The model under review builds one solid part; all positions refer to its coordinate system, in mm. Face numbers are marked on the shaded views. A direction names the side the tool comes from. Coordinates: 2 decimals unless noted, no trailing zeros. Write each loop counter-clockwise with the first axis right and the second up, starting at its lowest first coordinate (ties: lowest second). Pieces come first, ordered by that corner, then holes. Notation, with made-up numbers: (51, -23) - (97, -23) arc R13 ccw to (97, -12) - close; hole circle Ø6 at (34, -7.75). An arc over 180 degrees is marked (long way). Return JSON: item names as keys, results as strings. Group by question number.
(1) We need section C-C on y = -15.5. State the section outline as (x, z) points.
(2) We need section D-D on z = -16. State the section outline as (x, y) points.
(3) Draft analysis for pull direction X (two halves, no side actions). For the marked faces 4, 5, 6 and 7, state which applies: released by +X, released by -X, zero draft, split by the parting line, or undercut.
(4) We need section A-A on y = -43. State the section outline as (x, z) points.
(5) To check wall thickness, follow L1, parallel to Y at x = 0, z = -1.75; L2, parallel to Y at x = 34, z = 1.5; L3, parallel to Z at x = -31, y = -47. State the ranges of each line that lie inside material, in increasing order. Write a range as from..to.
(6) Tool access review of the marked faces 1, 2 and 3: name each direction out of +Z, -Z, +X, -X, +Y, -Y from which nothing blocks a thin tool from reaching the whole face with its end or side.
(7) For pin 1 Ø1.5 at (x, y) = (37, -30) entering from +Z; pin 2 Ø6 at (x, y) = (10.5, -14) entering from -Z; pin 3 Ø11.5 at (x, z) = (-12, 14) entering from -Y; pin 4 Ø17.5 at (x, y) = (0, -49.53) entering from +Z, all flat-tipped, find the tip position at first contact; note any pin that passes through.
(8) We need section B-B on x = 0. State the section outline as (y, z) points.
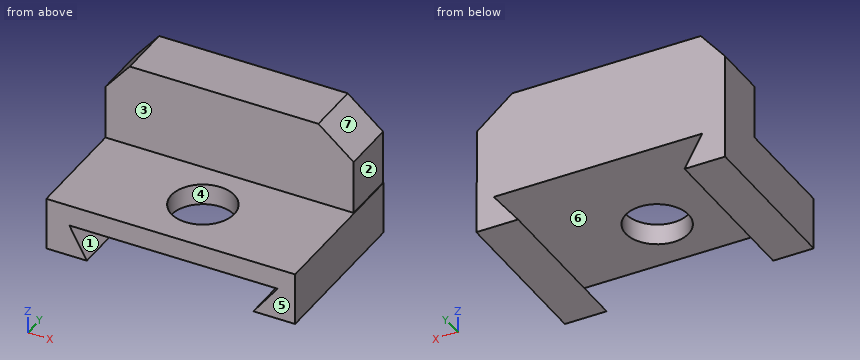
```python
from build123d import *

# Parameters (mm, degrees)
F1_DEPTH = 76.454
F3_DEPTH = 25.4
F4_R     = 14.704348
F5_DEPTH = 25.4


with BuildPart() as f1:
    # F0 (on Front) → F1 (new body)
    with BuildSketch(Plane.XZ):
        Polygon((57.71213, 0), (-58.586556, 0), (-58.586556, -24.629673), (-39.640658, -24.629673), (-47.801968, -9.764426), (49.55082, -9.764426), (38.183279, -24.629673), (57.71213, -24.629673), align=None)
    extrude(amount=F1_DEPTH)

    # F2 (on Front) → F3 (join)
    with BuildSketch(Plane.XZ):
        Polygon((-58.586556, 25.212623), (-58.586556, 0), (57.420652, 0), (57.420652, 25.212623), (40.911183, 38.911968), (-47.219016, 38.911968), align=None)
    extrude(amount=F3_DEPTH)

    # F4 (on Top) → F5 (cut)
    with BuildSketch(Plane.XY):
        with Locations((0, -49.532082)):
            Circle(F4_R)
    extrude(amount=-F5_DEPTH, mode=Mode.SUBTRACT)


solid = f1.part
```
Ans:
{
 "1": {"outline": "(-58.59, -24.63) - (-39.64, -24.63) - (-47.8, -9.76) - (49.55, -9.76) - (38.18, -24.63) - (57.71, -24.63) - (57.71, 0) - (57.42, 0) - (57.42, 25.21) - (40.91, 38.91) - (-47.22, 38.91) - (-58.59, 25.21) - close"},
 "2": {"outline": "(-58.59, -76.45) - (-44.38, -76.45) - (-44.38, 0) - (-58.59, 0) - close; (44.78, -76.45) - (57.71, -76.45) - (57.71, 0) - (44.78, 0) - close"},
 "3": {"face 4": "undercut", "face 5": "zero draft", "face 6": "undercut", "face 7": "released by +X"},
 "4": {"outline": "(-58.59, -24.63) - (-39.64, -24.63) - (-47.8, -9.76) - (-13.17, -9.76) - (-13.17, 0) - (-58.59, 0) - close; (13.17, -9.76) - (49.55, -9.76) - (38.18, -24.63) - (57.71, -24.63) - (57.71, 0) - (13.17, 0) - close"},
 "5": {"L1": "-76.45..-64.24, -34.83..0", "L2": "-25.4..0", "L3": "-9.76..0"},
 "6": {"face 1": "+Y, -Y", "face 2": "+Z, +X, +Y, -Y", "face 3": "+Z, +X, -X, -Y"},
 "7": {"pin 1": "z = 0", "pin 2": "z = -9.76", "pin 3": "y = -25.4", "pin 4": "through"},
 "8": {"outline": "(-76.45, -9.76) - (-64.24, -9.76) - (-64.24, 0) - (-76.45, 0) - close; (-34.83, -9.76) - (0, -9.76) - (0, 38.91) - (-25.4, 38.91) - (-25.4, 0) - (-34.83, 0) - close"}
}
